Part model, mm, in its own coordinate system. A direction names the side the tool comes from. Coordinates: 2 decimals unless noted, no trailing zeros. Loops run counter-clockwise (first coordinate to the right, second up) from the corner with the lowest first, then second, coordinate; pieces in that order, holes last. Notation, with made-up numbers: M 13,-25 L 25,-25 A24 ccw 25,-6 Z; hole C 89,19.25 d8. An arc over 180 degrees is marked long. Answer as CSV lines item,"result". Start each with the question number.
from build123d import *

# Parameters (mm, degrees)
BOSS_EXTRUDE1_DEPTH = 14
SKETCH2_W           = 14.019698715
SKETCH2_H           = 7.099583751
CUT_EXTRUDE1_DEPTH  = 1301.121764584
SKETCH4_R           = 2.54
CUT_EXTRUDE2_DEPTH  = 1238.809657762


with BuildPart() as part:
    # Sketch1 → Boss-Extrude1 (new body)
    with BuildSketch(Plane(origin=(0, 0, 0), x_dir=(1, 0, 0), z_dir=(0, 1, 0))):
        Polygon((-1237.710121457, -392.736417727), (-1237.710121457, -397.736417727), (-1212.710121457, -397.736417727), (-1212.710121457, -387.736417727), (-1237.710121457, -387.736417727), (-1237.710121457, -391.676417727), (-1229.710121457, -391.676417727), (-1229.710121457, -392.736417727), align=None)
    extrude(amount=-BOSS_EXTRUDE1_DEPTH)

    # Sketch2 → Cut-Extrude1 (cut, through all)
    with BuildSketch(Plane(origin=(0, 0, 0), x_dir=(1, 0, 0), z_dir=(0, 1, 0))):
        with Locations((-1219.719970814, -391.286209602)):
            Rectangle(SKETCH2_W, SKETCH2_H)
    extrude(amount=-CUT_EXTRUDE1_DEPTH, mode=Mode.SUBTRACT)

    # Sketch4 → Cut-Extrude2 (cut, through all)
    with BuildSketch(Plane(origin=(0, 0, 394.836001478), x_dir=(-1, 0, 0), z_dir=(0, 0, -1))):
        with Locations((1219.719970815, -7)):
            Circle(SKETCH4_R)
    extrude(amount=-CUT_EXTRUDE2_DEPTH, mode=Mode.SUBTRACT)


solid = part.part
Q1. Tool access for faces 5 (the face through (-1237.71, -7, 390)), 6 (the face through (-1234, -7, 391.676)), 7 (the face through (-1220, -10, 394.836)): list every direction of +Z, -Z, +X, -X, +Y, -Y with a clear straight run to the whole face (end or side of a thin tool).
Q2. Slice it at D-D, the plane y = -12.75. Write the cut outline in (x, z), and give its area (3 significant figures).
Q3. Flat gauge pins, fed straight in: P1, Ø7, axis at x = -1218, y = -6, coming from the -Z side; P2, Ø4, axis at x = -1223.5, z = 391, coming from the +Y side. Where does each tip first touch, or does it go through?
Q4. Slice it at C-C, the plane z = 394. Write the cut outline in (x, y), and give its area (3 significant figures).
Q5. Two-plate mould, pull along Z, no slides. Class faces 1 (the face through (-1234, -7, 392.736)), 2 (the face through (-1237.71, -7, 395)), 3 (the face through (-1225, -7, 397.736)), 4 (the face through (-1229.71, -7, 392)): +Z half, -Z half, draft (parallel to the pull), parting line (faces both ways), or undercut.
Q6. Slice it at B-B, the plane x = -1219.25. Write the cut outline in (y, z).
Q7. Slice it at A-A, the plane y = -7. Write the cut outline in (x, z), and give its area (3 significant figures).
Q8. Wall check: L1, parallel to Z at x = -1236.5, y = -7; L2, parallel to Z at x = -1223.25, y = -5.75; L3, parallel to X at y = -7.25, z = 390. Give the ranges that are in metal, low to high.
Solved:
1,face 5,"+Z, -Z, -X, +Y, -Y"
1,face 6,"-X, +Y, -Y"
1,face 7,"-Z, +X, +Y, -Y"
2,outline,"M -1237.71,387.74 L -1226.73,387.74 L -1226.73,394.84 L -1212.71,394.84 L -1212.71,397.74 L -1237.71,397.74 L -1237.71,392.74 L -1229.71,392.74 L -1229.71,391.68 L -1237.71,391.68 Z"
2,area,"142 mm2"
3,P1,"stops at z = 394.84"
3,P2,"passes through"
4,outline,"M -1237.71,-14 L -1226.73,-14 L -1226.73,0 L -1237.71,0 Z"
4,area,"154 mm2"
5,face 1,"undercut"
5,face 2,"draft"
5,face 3,"+Z half"
5,face 4,"undercut"
6,outline,"M -14,394.84 L -9.5,394.84 L -9.5,397.74 L -14,397.74 Z; M -4.5,394.84 L 0,394.84 L 0,397.74 L -4.5,397.74 Z"
7,outline,"M -1237.71,387.74 L -1226.73,387.74 L -1226.73,394.84 L -1222.26,394.84 L -1222.26,397.74 L -1237.71,397.74 L -1237.71,392.74 L -1229.71,392.74 L -1229.71,391.68 L -1237.71,391.68 Z; M -1217.18,394.84 L -1212.71,394.84 L -1212.71,397.74 L -1217.18,397.74 Z"
7,area,"127 mm2"
8,L1,"z = 387.74 to 391.68, 392.74 to 397.74"
8,L2,"z = 394.84 to 397.74"
8,L3,"x = -1237.71 to -1226.73"
